Source: three-view drawing plus pictorial views. Frame: mm from the lowest corner of the part. A direction names the side the tool comes from. Give positions to 0.01 mm unless a question says otherwise; leave off trailing zeros. Put each result on its own line as item: value. Start each with the question number.
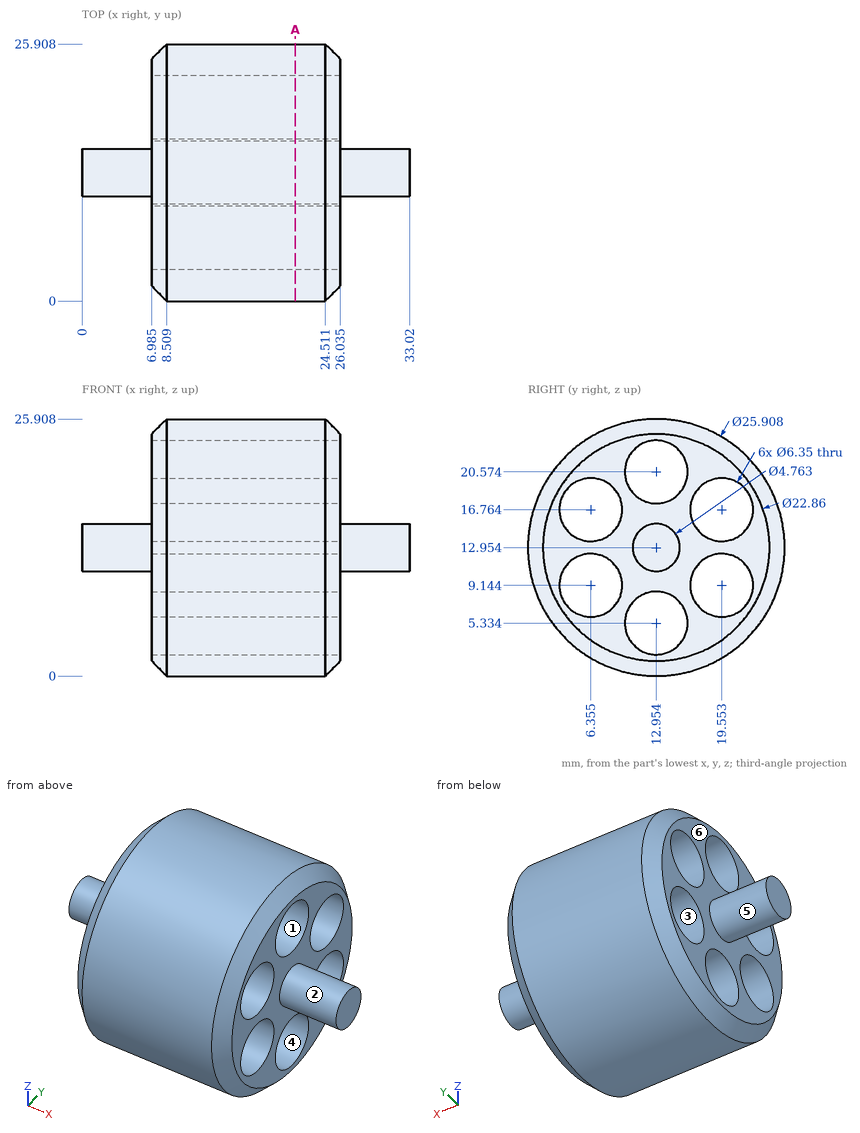
1. Contact query for flat-ended pins moving along their axis: pin 1 (1.5 mm diameter, centred on x = 10.5, y = 10.5, fed in from -Z); pin 2 (7.5 mm diameter, centred on y = 12.954, z = 5.334, fed in from +X) (1 decimal); pin 3 (10 mm diameter, centred on y = 6.35, z = 16.76, fed in from -X) (1 decimal); pin 4 (3 mm diameter, centred on y = 13.5, z = 15.5, fed in from +X). Output: stop coordinate, or through.
2. Pull-direction query (Z, two-part tool) for the marked faces 3, 4, 5 and 6; classes: released by +Z, released by -Z, zero draft, split by the parting line, or undercut.
3. Ray query, line 1 (Y direction, x = 24, z = 6.5) (1 decimal); line 2 (Z direction, x = 25.5, y = 7.25) (1 decimal); line 3 (Z direction, x = 19, y = 4.75) (1 decimal). Return the intervals inside material, ascending.
4. Set-up query: the marked faces 1 and 2. Return all of +Z, -Z, +X, -X, +Y, -Y with unobstructed straight access to the full face (end or side cutting, diameter ignored); none if empty.
5. Section A-A, the plane x = 21.5. State how many separate pieces and enclosed holes the cut face has, plus the area to 3 significant figures.
Results found:
1. pin 1: z = 0.11
1. pin 2: x = 26
1. pin 3: x = 7
1. pin 4: x = 33.02
2. face 3: undercut
2. face 4: undercut
2. face 5: split by the parting line
2. face 6: zero draft
3. line 1: 1.7 to 4.6, 8.1 to 10, 15.9 to 17.8, 21.3 to 24.2
3. line 2: 2.4 to 6.1, 12.2 to 13.7, 19.8 to 23.5
3. line 3: 2.9 to 6.4, 11.9 to 14, 19.5 to 23
4. face 1: +X, -X
4. face 2: +X
5. separate pieces: 1
5. enclosed holes: 6
5. area: 337 mm²
